Could you check a few things on this model? Use its own coordinates, in mm. Give positions to 0.01 mm unless a question says otherwise; leave off trailing zeros. Write each loop counter-clockwise with the first axis right and the second up, starting at its lowest first coordinate (ties: lowest second). Pieces come first, ordered by that corner, then holes. Notation, with made-up numbers: M 74.25,42 L 78.25,42 A11 ccw 78.25,47 Z; hole C 36.5,89 d7. An arc over 180 degrees is marked long. Use one line per item in the form item = value.
from build123d import *

# Parameters (mm, degrees)
SKETCH1_W            = 139.7
SKETCH1_H            = 12.7
BOSS_EXTRUDE1_DEPTH  = 6.35
SKETCH2_R            = 2.4511
CUT_EXTRUDE1_DEPTH   = 7.35
M3_CLEARANCE_HOLE1_D = 3.4


with BuildPart() as part:
    # Sketch1 → Boss-Extrude1 (new body)
    with BuildSketch(Plane.XY):
        Rectangle(SKETCH1_W, SKETCH1_H)
    extrude(amount=BOSS_EXTRUDE1_DEPTH)

    # Sketch2 → Cut-Extrude1 (cut, through all)
    with BuildSketch(Plane.XY.offset(6.35)):
        with Locations((0, 6.35)):
            Circle(SKETCH2_R)
        with Locations((5.334, 6.35)):
            Circle(SKETCH2_R)
        with Locations((10.668, 6.35)):
            Circle(SKETCH2_R)
        with Locations((16.002, 6.35)):
            Circle(SKETCH2_R)
        with Locations((21.336, 6.35)):
            Circle(SKETCH2_R)
        with Locations((26.67, 6.35)):
            Circle(SKETCH2_R)
        with Locations((32.004, 6.35)):
            Circle(SKETCH2_R)
        with Locations((37.338, 6.35)):
            Circle(SKETCH2_R)
        with Locations((42.672, 6.35)):
            Circle(SKETCH2_R)
        with Locations((48.006, 6.35)):
            Circle(SKETCH2_R)
        with Locations((53.34, 6.35)):
            Circle(SKETCH2_R)
        with Locations((58.674, 6.35)):
            Circle(SKETCH2_R)
        with Locations((-5.334, 6.35)):
            Circle(SKETCH2_R)
        with Locations((-10.668, 6.35)):
            Circle(SKETCH2_R)
        with Locations((-16.002, 6.35)):
            Circle(SKETCH2_R)
        with Locations((-21.336, 6.35)):
            Circle(SKETCH2_R)
        with Locations((-26.67, 6.35)):
            Circle(SKETCH2_R)
        with Locations((-32.004, 6.35)):
            Circle(SKETCH2_R)
        with Locations((-37.338, 6.35)):
            Circle(SKETCH2_R)
        with Locations((-42.672, 6.35)):
            Circle(SKETCH2_R)
        with Locations((-48.006, 6.35)):
            Circle(SKETCH2_R)
        with Locations((-53.34, 6.35)):
            Circle(SKETCH2_R)
        with Locations((-58.674, 6.35)):
            Circle(SKETCH2_R)
    extrude(amount=-CUT_EXTRUDE1_DEPTH, mode=Mode.SUBTRACT)

    # M3 Clearance Hole1 (through all)
    with Locations(Plane(origin=(0, -6.35, 0), x_dir=(-1, 0, 0), z_dir=(0, -1, 0))):
        with Locations((65.0875, -3.175)):
            m3_clearance_hole1 = Hole(M3_CLEARANCE_HOLE1_D / 2)

    # Mirror1: M3 Clearance Hole1 across plane
    add(m3_clearance_hole1.mirror(Plane(origin=(0, 0, 0), x_dir=(0, 0, 1), z_dir=(1, 0, 0))), mode=Mode.SUBTRACT)


solid = part.part
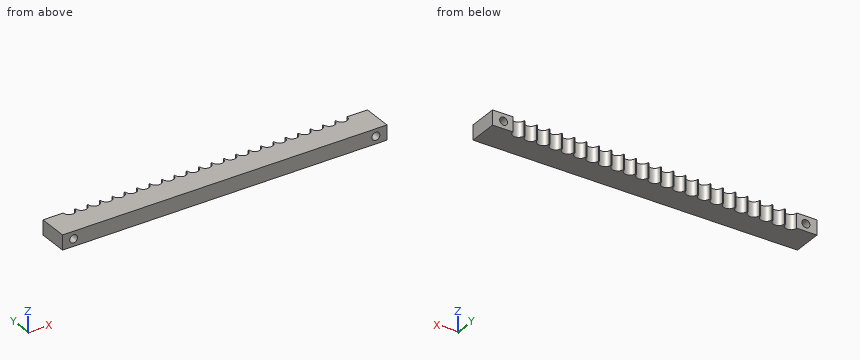
1) I want a section at C-C, the plane x = 17. Please give me the cut outline in (y, z).
Checked values:
outline = M -6.35,0 L 4.11,0 L 4.11,6.35 L -6.35,6.35 Z
2) I want a section at A-A, the plane y = -4.25. Count the separate pieces of the cut face and the enclosed holes in it, plus the area to 3 significant figures.
Checked values:
separate_pieces = 1
enclosed_holes = 2
area = 869 mm2
3) I want a section at B-B, the plane x = 0. Please give me the cut outline in (y, z), plus the area to 3 significant figures.
Checked values:
outline = M -6.35,0 L 3.9,0 L 3.9,6.35 L -6.35,6.35 Z
area = 65.1 mm2
4) If I drill on L1, parallel to X at y = 0, z = 2.25; L2, parallel to X at y = -3, z = 2.75; L3, parallel to Y at x = 59, z = 1.75, over which ranges is the centre line in solid material (lowest first)?
Checked values:
L1 = -69.85 to -66.51, -63.66 to 63.66, 66.51 to 69.85
L2 = -69.85 to -66.73, -63.44 to 63.44, 66.73 to 69.85
L3 = -6.35 to 3.92
